Build history of the part. All positions in model axes, mm. Round coordinates to 2 decimals unless told otherwise and drop trailing zeros.
1) Wall check: probe 1 along X at (y, z) = (-49, 0.45); probe 2 along X at (y, z) = (-47.5, 0.35); probe 3 along X at (y, z) = (52, 0.3). Give the ranges that are in metal, low to high.
2) Saw through at A-A (z = 1.45). State how many separate pieces and enclosed holes the cut face has, plus the area to 3 significant figures.
3) Flat gauge pin, fed straight in: pin 1 (1 mm diameter, centred on y = 42, z = 0.5, fed in from +X). Where does the tip first touch, or does it go through?
from build123d import *

# Parameters (mm, degrees)
SKETCH3_W               = 200
SKETCH3_H               = 140
BOSS_EXTRUDE1_DEPTH     = 2
SKETCH7_R               = 1.5
CUT_EXTRUDE1_DEPTH      = 123.081939696
SKETCH8_R               = 1.5
CUT_EXTRUDE2_DEPTH      = 123.081939696
CUT_EXTRUDE5_START      = -2
CUT_EXTRUDE5_DEPTH      = 2
CUT_EXTRUDE6_DEPTH      = 123.081939837
CUT_EXTRUDE6_DEPTH_BACK = 123.081939837


# Read off the part's stored shape, not the designer's step: Cut-Extrude5
with BuildPart() as part:
    # Sketch3 → Boss-Extrude1 (new body)
    with BuildSketch(Plane.XY):
        Rectangle(SKETCH3_W, SKETCH3_H)
    extrude(amount=BOSS_EXTRUDE1_DEPTH)

    # Sketch7 → Cut-Extrude1 (cut, through all)
    with BuildSketch(Plane.XY.offset(2)):
        with Locations((-80, -44)):
            Circle(SKETCH7_R)
        with Locations((-51, -50)):
            Circle(SKETCH7_R)
        with Locations((-51, -38)):
            Circle(SKETCH7_R)
        with Locations((-51, -44)):
            Circle(SKETCH7_R)
        with Locations((-80, -50)):
            Circle(SKETCH7_R)
        with Locations((-80, -38)):
            Circle(SKETCH7_R)
    extrude(amount=-CUT_EXTRUDE1_DEPTH, mode=Mode.SUBTRACT)

    # Sketch8 → Cut-Extrude2 (cut, through all)
    with BuildSketch(Plane.XY.offset(2)):
        with Locations((-80, 50.001919615)):
            Circle(SKETCH8_R)
        with Locations((-80, 44.001919615)):
            Circle(SKETCH8_R)
        with Locations((-80, 38.001919615)):
            Circle(SKETCH8_R)
        with Locations((-51, 50.001919615)):
            Circle(SKETCH8_R)
        with Locations((-51, 44.001919615)):
            Circle(SKETCH8_R)
        with Locations((-51, 38.001919615)):
            Circle(SKETCH8_R)
        with Locations((80, 50.001919615)):
            Circle(SKETCH8_R)
        with Locations((80, 44.001919615)):
            Circle(SKETCH8_R)
        with Locations((80, 38.001919615)):
            Circle(SKETCH8_R)
        with Locations((51, 50.001919615)):
            Circle(SKETCH8_R)
        with Locations((51, 44.001919615)):
            Circle(SKETCH8_R)
        with Locations((51, 38.001919615)):
            Circle(SKETCH8_R)
        with Locations((51, -38)):
            Circle(SKETCH8_R)
        with Locations((51, -44)):
            Circle(SKETCH8_R)
        with Locations((51, -50)):
            Circle(SKETCH8_R)
        with Locations((80, -38)):
            Circle(SKETCH8_R)
        with Locations((80, -44)):
            Circle(SKETCH8_R)
        with Locations((80, -50)):
            Circle(SKETCH8_R)
    extrude(amount=-CUT_EXTRUDE2_DEPTH, mode=Mode.SUBTRACT)

    # Cut-Extrude5 outline → Cut-Extrude5 (cut)
    with BuildSketch(Plane.XY.offset(2).offset(CUT_EXTRUDE5_START)):
        with BuildLine():
            add(Edge.make_bspline(
                [(-100, 0), (-100, -35), (-80, -70)],
                knots=[0.5, 0.5, 0.5, 1, 1, 1], degree=2))
            Line((-100, 0), (-100, -70))
            Line((-100, -70), (-80, -70))
        make_face()
        with BuildLine():
            add(Edge.make_bspline(
                [(-80, 70), (-100, 35), (-100, 0)],
                knots=[0, 0, 0, 0.5, 0.5, 0.5], degree=2))
            Line((-80, 70), (-100, 70))
            Line((-100, 70), (-100, 0))
        make_face()
    extrude(amount=CUT_EXTRUDE5_DEPTH, mode=Mode.SUBTRACT)

    # Sketch16 → Cut-Extrude6 (cut, two sides: drawn at the far end of the back side and taken through both)
    with BuildSketch(Plane.XY.offset(2).offset(-CUT_EXTRUDE6_DEPTH_BACK)):
        with BuildLine():
            Line((100, 70), (80, 70))
            add(Edge.make_bspline(
                [(80, 70), (100.000000027, 34.999999953), (100, -9.3e-08)],
                knots=[0, 0, 0, 0.500000001, 0.500000001, 0.500000001], degree=2))
            Line((100, -9.3e-08), (100, 70))
        make_face()
        with BuildLine():
            Line((100, -70), (100, -9.3e-08))
            add(Edge.make_bspline(
                [(100, -9.3e-08), (99.999999973, -35.000000047), (80, -70)],
                knots=[0.500000001, 0.500000001, 0.500000001, 1, 1, 1], degree=2))
            Line((80, -70), (100, -70))
        make_face()
    extrude(amount=CUT_EXTRUDE6_DEPTH + CUT_EXTRUDE6_DEPTH_BACK, mode=Mode.SUBTRACT)


solid = part.part
Evaluation:
1. probe 1: x = -90.2 to -81.12, -78.88 to -52.12, -49.88 to 49.88, 52.12 to 78.88, 81.12 to 90.2
1. probe 2: x = -90.79 to 90.79
1. probe 3: x = -88.96 to 88.96
2. separate pieces: 1
2. enclosed holes: 24
2. area: 26,000 mm2
3. pin 1: stops at x = 92.97
